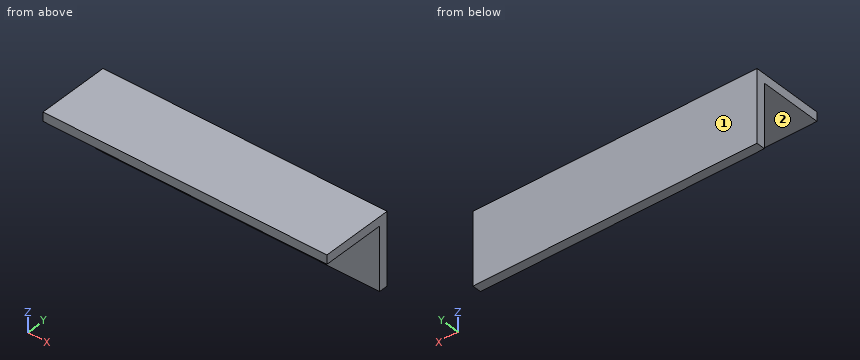
Autodesk Inventor part; units mm, degrees
ref_plane "YZ Plane" through (0, 0, 0) normal (1, 0, 0) x (0, 1, 0)
ref_plane "XZ Plane" through (0, 0, 0) normal (0, 1, 0) x (-1, 0, 0)
ref_plane "XY Plane" through (0, 0, 0) normal (0, 0, 1) x (1, 0, 0)
sketch "Sketch1" plane through (0, 0, 0) normal (1, 0, 0) x (0, 1, 0)
  line L0 (0, 0) -> (-25.4, 0)
  line L1 (-25.4, 0) -> (-25.4, -3.175)
  line L2 (-25.4, -3.175) -> (0, -3.175)
  line L3 (0, -3.175) -> (0, 0)
  line L4 (0, 0) -> (-3.175, 0)
  line L5 (-3.175, 0) -> (-3.175, -25.4)
  line L6 (-3.175, -25.4) -> (0, -25.4)
  line L7 (0, -25.4) -> (0, 0)
  point P0 (-3.175, -3.175)
  dimension "d0" = 3.175
  dimension "d1" = 25.4
extrude "Extrusion1" add sketch "Sketch1" along normal blind 100
properties part number "SOPORTE_CANALETA_PRINCIPAL" material "Steel, Mild, Welded"
Could you check a few things on this model? Use its own coordinates, in mm. Face numbers are marked on the shaded views. A direction names the side the tool comes from. Round coordinates to 2 decimals unless told otherwise and drop trailing zeros. Write each loop counter-clockwise with the first axis right and the second up, starting at its lowest first coordinate (ties: lowest second). Pieces come first, ordered by that corner, then holes.
(1) If I drill on probe 1 along Z at (x, y) = (96.5, -15) (3 decimals), over which ranges is the centre line in solid material (lowest first)?
Findings below:
probe 1: z = -3.175 to 0
(2) Suppose I cut it at B-B on y = -11.5. Write out the boundary of the cut face in (x, z) (3 decimals), and give its area (4 significant figures).
Findings below:
outline: (0, -3.175) - (100, -3.175) - (100, 0) - (0, 0) - close
area: 317.5 mm2
(3) Which directions (+Z, -Z, +X, -X, +Y, -Y) give clear straight access to the entire face, cutting with the end or side of a thin tool? Please do the marked faces 1 and 2.
Findings below:
face 1: +Z, -Z, +X, -X, +Y
face 2: -Z, +X, -X, -Y
(4) For pin 1 (11 mm diameter, centred on x = 70.5, z = -11, fed in from -Y) (3 decimals); pin 2 (6 mm diameter, centred on x = 47.5, y = -15.5, fed in from -Z) (3 decimals), each with a flat end and sliding along its axis, tell me the tip position at first contact or that it passes through.
Findings below:
pin 1: stops at y = -3.175
pin 2: stops at z = -3.175
(5) Suppose I cut it at A-A on x = 34.5. Write out the boundary of the cut face in (y, z) (3 decimals), and give its area (3 significant figures).
Findings below:
outline: (-25.4, -3.175) - (-3.175, -3.175) - (-3.175, -25.4) - (0, -25.4) - (0, 0) - (-25.4, 0) - close
area: 151 mm2
